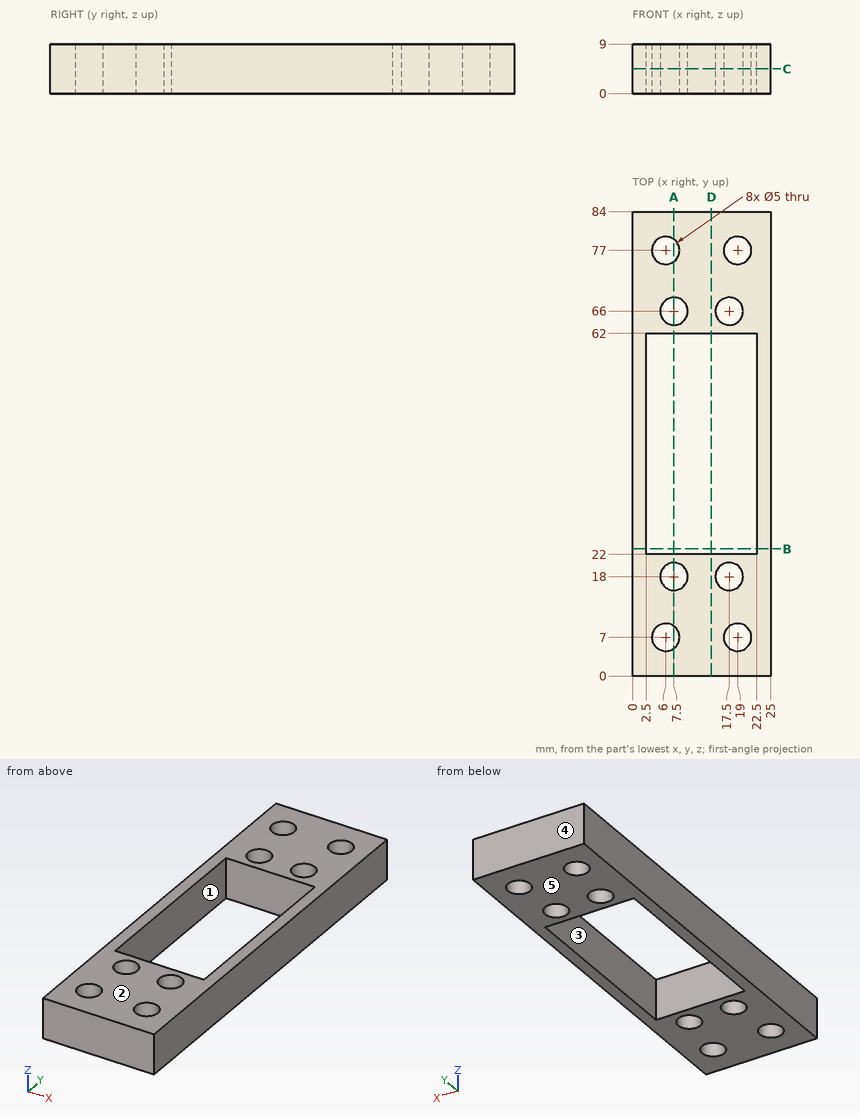
Print and shaded views of the part. All mm, measured from the part's lowest x, y and z. A direction names the side the tool comes from. Give positions to 0.01 mm unless a question says otherwise; leave off trailing zeros. Write each loop counter-clockwise with the first axis right and the second up, starting at its lowest first coordinate (ties: lowest second). Pieces come first, ordered by that corner, then holes. Notation, with made-up numbers: (39.5, 55.5) - (79.5, 55.5) arc R10 cw to (79.5, 60.5) - close; hole circle Ø6 at (34, -11). An arc over 180 degrees is marked (long way). Put each result on its own line as item: value.
(1) Pull direction Y, two halves, no side cores. Call the marked faces 3, 4 and 5: released by +Y, released by -Y, zero draft, split by the parting line, or undercut.
Working result:
face 3: undercut
face 4: released by +Y
face 5: zero draft
(2) Wall check: L1, parallel to Y at x = 7.5, z = 5.25; L2, parallel to X at y = 26, z = 1.25; L3, parallel to Y at x = 10.5, z = 2.25. Give the ranges that are in metal, low to high.
Working result:
L1: 0 to 5, 9 to 15.5, 20.5 to 22, 62 to 63.5, 68.5 to 75, 79 to 84
L2: 0 to 2.5, 22.5 to 25
L3: 0 to 22, 62 to 84
(3) Drop a flat-ended pin along its axis: pin 1 Ø6.5 at (x, y) = (19, 7) entering from +Z. Give the stop position or say it passes through.
Working result:
pin 1: z = 9
(4) Saw through at D-D (x = 14.25). List the corners of the cut face in (y, z).
Working result:
outline: (0, 0) - (22, 0) - (22, 9) - (0, 9) - close; (62, 0) - (84, 0) - (84, 9) - (62, 9) - close
(5) Tool access for the marked faces 1 and 2: list every direction of +Z, -Z, +X, -X, +Y, -Y with a clear straight run to the whole face (end or side of a thin tool).
Working result:
face 1: +Z, -Z
face 2: +Z, +X, -X, +Y, -Y
(6) Saw through at A-A (x = 7.5). List the corners of the cut face in (y, z).
Working result:
outline: (0, 0) - (5, 0) - (5, 9) - (0, 9) - close; (9, 0) - (15.5, 0) - (15.5, 9) - (9, 9) - close; (20.5, 0) - (22, 0) - (22, 9) - (20.5, 9) - close; (62, 0) - (63.5, 0) - (63.5, 9) - (62, 9) - close; (68.5, 0) - (75, 0) - (75, 9) - (68.5, 9) - close; (79, 0) - (84, 0) - (84, 9) - (79, 9) - close
(7) Saw through at C-C (z = 4.5). Count the separate pieces of the cut face and the enclosed holes in it, then the cut area to 3 significant figures.
Working result:
separate pieces: 1
enclosed holes: 9
area: 1,140 mm^2
(8) Saw through at B-B (y = 23). List the corners of the cut face in (x, z), then the cut area to 3 significant figures.
Working result:
outline: (0, 0) - (2.5, 0) - (2.5, 9) - (0, 9) - close; (22.5, 0) - (25, 0) - (25, 9) - (22.5, 9) - close
area: 45.0 mm^2
